Source: CAD feature listing. Evaluate the final solid. Frame: model axes, mm. A direction names the side the tool comes from. Round coordinates to 2 decimals unless told otherwise and drop trailing zeros. Write each loop counter-clockwise with the first axis right and the second up, starting at its lowest first coordinate (ties: lowest second). Pieces come first, ordered by that corner, then holes. Notation, with made-up numbers: (59.5, 17) -> (82.5, 17) arc R6 ccw to (82.5, 24) -> close; hole circle Ø9 at (-36, 58). An arc over 180 degrees is marked (long way). Return JSON: item names as keys, results as strings. Group by question number.
from build123d import *

# Parameters (mm, degrees)
SKETCH1_R      = 7.25
EXTRUDE1_DEPTH = 5


with BuildPart() as part:
    # Sketch1 → Extrude1 (new body)
    with BuildSketch(Plane.XY):
        with BuildLine():
            Line((21.155672998, -1), (22.078640359, -1))
            ThreePointArc((22.078640359, -1), (22.661735548, -1.18759616), (23.026057901, -1.68))
            ThreePointArc((23.026057901, -1.68), (33.25, 0), (23.026057901, 1.68))
            ThreePointArc((23.026057901, 1.68), (22.661735548, 1.18759616), (22.078640359, 1))
            Line((22.078640359, 1), (21.2294652, 1))
            ThreePointArc((21.2294652, 1), (20.50121081, 1.314693102), (20.231309687, 2.060708911))
            ThreePointArc((20.231309687, 2.060708911), (26.941055993, 10.661478857), (37.377512662, 7.48747329))
            ThreePointArc((37.377512662, 7.48747329), (39.325417254, 3.966727118), (40, 0))
            Line((40, 0), (40, -35.220781011))
            ThreePointArc((40, -35.220781011), (40.315942047, -38.231179655), (41.25, -41.110390505))
            ThreePointArc((41.25, -41.110390505), (35.920463529, -59.145627093), (17.267456033, -56.75))
            ThreePointArc((17.267456033, -56.75), (12.403259363, -53.240569394), (6.534912066, -52))
            Line((6.534912066, -52), (-6.534912066, -52))
            ThreePointArc((-6.534912066, -52), (-12.403259363, -53.240569394), (-17.267456033, -56.75))
            ThreePointArc((-17.267456033, -56.75), (-35.920463529, -59.145627093), (-41.25, -41.110390505))
            ThreePointArc((-41.25, -41.110390505), (-40.315942047, -38.231179655), (-40, -35.220781011))
            Line((-40, -35.220781011), (-40, 0))
            ThreePointArc((-40, 0), (-39.325417254, 3.966727118), (-37.377512662, 7.48747329))
            ThreePointArc((-37.377512662, 7.48747329), (-26.941055993, 10.661478857), (-20.231309687, 2.060708911))
            ThreePointArc((-20.231309687, 2.060708911), (-20.50121081, 1.314693102), (-21.2294652, 1))
            Line((-21.2294652, 1), (-22.078640359, 1))
            ThreePointArc((-22.078640359, 1), (-22.661735548, 1.18759616), (-23.026057901, 1.68))
            ThreePointArc((-23.026057901, 1.68), (-33.25, 0), (-23.026057901, -1.68))
            ThreePointArc((-23.026057901, -1.68), (-22.661735548, -1.18759616), (-22.078640359, -1))
            Line((-22.078640359, -1), (-21.155672998, -1))
            ThreePointArc((-21.155672998, -1), (-20.482663952, -1.26036575), (-20.160111916, -1.905882353))
            ThreePointArc((-20.160111916, -1.905882353), (-14.318912319, -14.318912319), (-1.905882353, -20.160111916))
            ThreePointArc((-1.905882353, -20.160111916), (-1.26036575, -20.482663952), (-1, -21.155672998))
            Line((-1, -21.155672998), (-1, -22.078640359))
            ThreePointArc((-1, -22.078640359), (-1.18759616, -22.661735548), (-1.68, -23.026057901))
            ThreePointArc((-1.68, -23.026057901), (0, -33.25), (1.68, -23.026057901))
            ThreePointArc((1.68, -23.026057901), (1.18759616, -22.661735548), (1, -22.078640359))
            Line((1, -22.078640359), (1, -21.155672998))
            ThreePointArc((1, -21.155672998), (1.26036575, -20.482663952), (1.905882353, -20.160111916))
            ThreePointArc((1.905882353, -20.160111916), (14.318912319, -14.318912319), (20.160111916, -1.905882353))
            ThreePointArc((20.160111916, -1.905882353), (20.482663952, -1.26036575), (21.155672998, -1))
        make_face()
        with Locations((28, -47)):
            Circle(SKETCH1_R, mode=Mode.SUBTRACT)
        with Locations((-28, -47)):
            Circle(SKETCH1_R, mode=Mode.SUBTRACT)
    extrude(amount=EXTRUDE1_DEPTH)


solid = part.part
Item 1: Material intervals for probe 1 along X at (y, z) = (-28, 4.05); probe 2 along Y at (x, z) = (-28, 2.85); probe 3 along X at (y, z) = (-3.5, 2.25), sorted ascending.
Item 2: Cut plane B-B on x = -28. Output: boundary loops of the cut face in (y, z).
Item 3: Cut plane D-D on z = 1.55. Give the number of separate pieces and of enclosed holes in the cut face, and give its area (3 significant figures).
Item 4: Set-up query: faces 4 (the cylindrical face through (-39.344, 3.913, 2.465)), 5 (the cylindrical face through (22.247, -51.412, 2.465)), 6 (the cylindrical face through (14.18, -14.457, 2.465)), 7 (the flat face through (0, -52, 2)), 8 (the flat face through (40, -17, 2)). Return all of +Z, -Z, +X, -X, +Y, -Y with unobstructed straight access to the full face (end or side cutting, diameter ignored); none if empty.
Item 5: Cut plane A-A on y = -28. Output: boundary loops of the cut face in (x, z), and give its area (4 significant figures).
Item 6: First-contact query: pin 1 Ø0.5 at (y, z) = (-21.5, 2.5) entering from +X; pin 2 Ø0.9 at (x, z) = (-21.5, 3.5) entering from -Y; pin 3 Ø0.7 at (x, z) = (-21.5, 3) entering from +Y; pin 4 Ø8.5 at (x, y) = (-28, 0) entering from -Z. Flat tips, straight axial feed; report the tip coordinate or a pass-through.
Item 7: Cut plane C-C on y = -47. Output: boundary loops of the cut face in (x, z).
Item 8: Pull-direction query (X, two-part tool) for faces 1 (the flat face through (-9, -33, 5)), 2 (the flat face through (-40, -18, 2)), 3 (the cylindrical face through (-14.457, -14.18, 2.465)); classes: +X half, -X half, draft (parallel to the pull), parting line (faces both ways), or undercut.
Here are the results:
{
 "1": {"probe 1": "x = -40 to -5.25, 5.25 to 40", "probe 2": "y = -61.5 to -54.25, -39.75 to -5.25, 5.25 to 10.93", "probe 3": "x = -40 to -31.91, -24.09 to -19.95, 19.95 to 24.09, 31.91 to 40"},
 "2": {"outline": "(-61.5, 0) -> (-54.25, 0) -> (-54.25, 5) -> (-61.5, 5) -> close; (-39.75, 0) -> (-5.25, 0) -> (-5.25, 5) -> (-39.75, 5) -> close; (5.25, 0) -> (10.93, 0) -> (10.93, 5) -> (5.25, 5) -> close"},
 "3": {"separate pieces": "1", "enclosed holes": "2", "area": "3,700 mm^2"},
 "4": {"face 4": "+Z, -Z, -X, +Y", "face 5": "+Z, -Z", "face 6": "+Z, -Z, +Y", "face 7": "+Z, -Z, -Y", "face 8": "+Z, -Z, +X, +Y"},
 "5": {"outline": "(-40, 0) -> (-5.25, 0) -> (-5.25, 5) -> (-40, 5) -> close; (5.25, 0) -> (40, 0) -> (40, 5) -> (5.25, 5) -> close", "area": "347.5 mm^2"},
 "6": {"pin 1": "stops at x = 40", "pin 2": "stops at y = -60.18", "pin 3": "stops at y = 6.85", "pin 4": "passes through"},
 "7": {"outline": "(-42.5, 0) -> (-35.25, 0) -> (-35.25, 5) -> (-42.5, 5) -> close; (-20.75, 0) -> (20.75, 0) -> (20.75, 5) -> (-20.75, 5) -> close; (35.25, 0) -> (42.5, 0) -> (42.5, 5) -> (35.25, 5) -> close"},
 "8": {"face 1": "draft", "face 2": "-X half", "face 3": "undercut"}
}
